Here's how the part is built. I have some questions about the finished solid (model axes, mm). Coordinates: 2 decimals unless noted, no trailing zeros. Write each loop counter-clockwise with the first axis right and the second up, starting at its lowest first coordinate (ties: lowest second). Pieces come first, ordered by that corner, then holes. Notation, with made-up numbers: (10.5, -36) -> (19.5, -36) arc R20 cw to (19.5, -3) -> close; hole circle Ø7 at (80.5, -2). An arc over 180 degrees is marked (long way). Use a Markdown table: item, result. Add a question column.
Item 1: If I drill on line 1 along Z through (x, y) = (13.25, -56.5); line 2 along X through (y, z) = (-376, 993); line 3 along Z through (x, y) = (10.75, -353) (3 decimals), over which ranges is the centre line in solid material (lowest first)? Write a range as from..to.
Item 2: Will these pins go through, and if not, where does the flat tip stop? pin 1 Ø9 at (y, z) = (-291, 988) entering from +X; pin 2 Ø8 at (y, z) = (-161, 729) entering from -X; pin 3 Ø9 at (x, y) = (10, -368) entering from -Z (3 decimals).
Item 3: Imagine slicing it at A-A, the plane y = -377.5. Write out the boundary of the cut face in (x, z) (1 decimal).
```python
from build123d import *

# Parameters (mm, degrees)
F0_W     = 18.25625
F0_H     = 2064.54375
F1_DEPTH = 406.4
F3_DEPTH = 406.4
F4_W     = 55.88
F4_H     = 19.685
F5_DEPTH = 25.4


with BuildPart() as f1:
    # F0 (on Front) → F1 (new body)
    with BuildSketch(Plane.XZ):
        with Locations((9.128125, 1032.271875)):
            Rectangle(F0_W, F0_H)
    extrude(amount=F1_DEPTH)

    # F2 (on face) → F3 (cut)
    with BuildSketch(Plane.XZ.offset(406.4)):
        Polygon((11.90625, 73.03135), (18.25625, 73.03135), (18.25625, 91.2876), (18.25625, 91.29395), (11.90625, 91.29395), align=None)
        Polygon((11.90625, 980.28125), (18.25625, 980.28125), (18.25625, 995.793984), (18.25625, 998.5375), (11.90625, 998.5375), align=None)
    extrude(amount=-F3_DEPTH, mode=Mode.SUBTRACT)

    # F4 (on face) → F5 (cut)
    with BuildSketch(Plane(origin=(0, 0, 0), x_dir=(0, -1, 0), z_dir=(-1, 0, 0))):
        with Locations((378.46, 9.8425)):
            Rectangle(F4_W, F4_H)
    extrude(amount=-F5_DEPTH, mode=Mode.SUBTRACT)


solid = f1.part
```
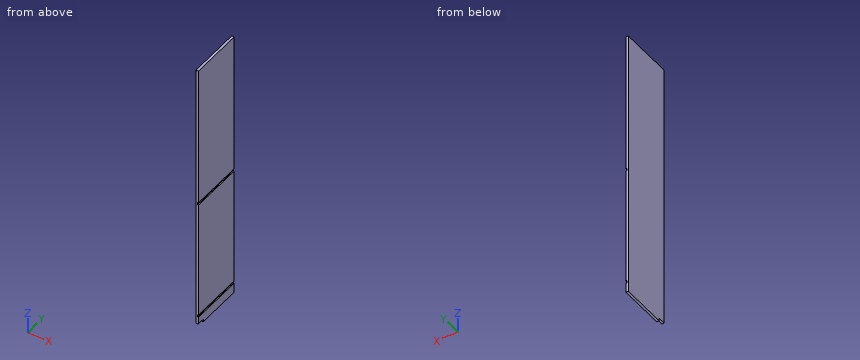
Ans:
| question | item | result |
|---|---|---|
| 1 | line 1 | z = 0..73.03, 91.29..980.28, 998.54..2064.54 |
| 1 | line 2 | x = 0..11.91 |
| 1 | line 3 | z = 19.685..2064.544 |
| 2 | pin 1 | stops at x = 11.91 |
| 2 | pin 2 | stops at x = 0 |
| 2 | pin 3 | stops at z = 19.685 |
| 3 | outline | (0, 19.7) -> (18.3, 19.7) -> (18.3, 73) -> (11.9, 73) -> (11.9, 91.3) -> (18.3, 91.3) -> (18.3, 980.3) -> (11.9, 980.3) -> (11.9, 998.5) -> (18.3, 998.5) -> (18.3, 2064.5) -> (0, 2064.5) -> close |
